Geometry check sheet. Reference: the model listing, model coordinates, mm. Face numbers are marked on the shaded views. A direction names the side the tool comes from. Give positions to 0.01 mm unless a question says otherwise; leave off trailing zeros. Write each loop counter-clockwise with the first axis right and the second up, starting at its lowest first coordinate (ties: lowest second). Pieces come first, ordered by that corner, then holes. Notation, with made-up numbers: (75, 72.25) - (117, 72.25) arc R27 cw to (117, 103.25) - close; hole circle Ø10 at (17, 81). An arc over 180 degrees is marked (long way). Write item = value, one per line. Start each with the question number.
(1) Section check B-B, the plane y = -12.85. Enter the section's corners in (x, z).
(2) Access from +Z, -Z, +X, -X, +Y, -Y to the whole of each face (thin tool, end or side, straight path). Record for the marked faces 1 and 2.
(3) Draft check along Y on the marked faces 3, 4 and 5. Enter one of: pulls with the +Y half, pulls with the -Y half, needs draft (parallel to the pull), parting line crosses it, or undercut.
(4) Thickness scan on L1, parallel to Y at x = 0, z = -0.95; L2, parallel to Z at x = 12, y = -9.5; L3, parallel to Y at x = 12.85, z = -1.2. Record the ranges inside material, lowest first.
(5) Section check C-C, the plane z = 5. Enter the section's corners in (x, y).
(6) Section check D-D, the plane y = 3.75. Enter the section's corners in (x, z), plus the area to 3 significant figures.
(7) Depth check by flat-ended pin: pin 1 Ø1.8 at (y, z) = (3, 2) entering from +X; pin 2 Ø5 at (y, z) = (-12.5, 3) entering from -X; pin 3 Ø1.5 at (y, z) = (-6, 3.5) entering from -X; pin 4 Ø2 at (y, z) = (1, 4) entering from -X. Enter the tip coordinate at first touch or a pass-through.
(8) Section check A-A, the plane x = 0. Enter the section's corners in (y, z).
```python
from build123d import *

# Parameters (mm, degrees)
F1_DEPTH = 2.5
F2_DEPTH = 7.5
F3_SIZE  = 0.5
F4_R     = 1.4
F5_DEPTH = 25


with BuildPart() as f1:
    # F0 (on Top) → F1 (new body)
    with BuildSketch(Plane.XY):
        with BuildLine():
            Line((11.83183, 11.514682), (8.85, 6.35))
            Line((8.85, 6.35), (8.85, 0))
            ThreePointArc((8.85, 0), (0, -8.85), (-8.85, 0))
            Line((-8.85, 0), (-8.85, 6.35))
            Line((-8.85, 6.35), (-11.83183, 11.514682))
            ThreePointArc((-11.83183, 11.514682), (0, -16.51), (11.83183, 11.514682))
        make_face()
        with BuildLine():
            Line((6.35, 2.019873), (6.35, 0))
            ThreePointArc((6.35, 0), (0, -6.35), (-6.35, 0))
            Line((-6.35, 0), (-6.35, 2.019873))
            Line((-6.35, 2.019873), (-8.85, 6.35))
            Line((-8.85, 6.35), (-8.85, 0))
            ThreePointArc((-8.85, 0), (0, -8.85), (8.85, 0))
            Line((8.85, 0), (8.85, 6.35))
            Line((8.85, 6.35), (6.35, 2.019873))
        make_face()
    extrude(amount=-F1_DEPTH)

    # F0 (on Top) → F2 (join)
    with BuildSketch(Plane.XY):
        with BuildLine():
            Line((6.35, 2.019873), (6.35, 0))
            ThreePointArc((6.35, 0), (0, -6.35), (-6.35, 0))
            Line((-6.35, 0), (-6.35, 2.019873))
            Line((-6.35, 2.019873), (-8.85, 6.35))
            Line((-8.85, 6.35), (-8.85, 0))
            ThreePointArc((-8.85, 0), (0, -8.85), (8.85, 0))
            Line((8.85, 0), (8.85, 6.35))
            Line((8.85, 6.35), (6.35, 2.019873))
        make_face()
    extrude(amount=F2_DEPTH)

    # F3
    f3_edges = [f1.edges().sort_by_distance(p)[0] for p in [
        (-8.85, 6.35, 3.75),
        (8.85, 6.35, 3.75),
    ]]
    chamfer(f3_edges, length=F3_SIZE)

    # F4 (on face) → F5 (cut)
    with BuildSketch(Plane.XY):
        with Locations((-12.85, 0)):
            Circle(F4_R)
        with Locations((12.85, 0)):
            Circle(F4_R)
        with Locations((0, -12.85)):
            Circle(F4_R)
    extrude(amount=-F5_DEPTH, mode=Mode.SUBTRACT)


solid = f1.part
```
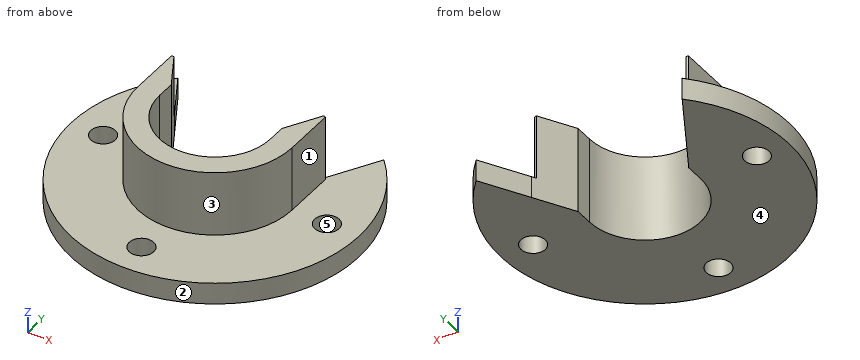
Model answer:
q1.outline = (-10.37, -2.5) - (-1.4, -2.5) - (-1.4, 0) - (-10.37, 0) - close; (1.4, -2.5) - (10.37, -2.5) - (10.37, 0) - (1.4, 0) - close
q2.face_1 = +Z, +X, +Y, -Y
q2.face_2 = +Z, -Z
q3.face_3 = pulls with the -Y half
q3.face_4 = needs draft
q3.face_5 = undercut
q4.L1 = -16.51 to -14.25, -11.45 to -6.35
q4.L2 = -2.5 to 0
q4.L3 = -10.37 to -1.4, 1.4 to 10.37
q5.outline = (-8.85, 0) arc R8.85 ccw to (8.85, 0) - (8.85, 5.85) - (8.6, 5.92) - (6.35, 2.02) - (6.35, 0) arc R6.35 cw to (-6.35, 0) - (-6.35, 2.02) - (-8.6, 5.92) - (-8.85, 5.85) - close
q6.outline = (-16.08, -2.5) - (-7.35, -2.5) - (-7.35, 7.5) - (-8.85, 7.5) - (-8.85, 0) - (-16.08, 0) - close; (7.35, -2.5) - (16.08, -2.5) - (16.08, 0) - (8.85, 0) - (8.85, 7.5) - (7.35, 7.5) - close
q6.area = 66.2 mm²
q7.pin_1 = 8.85
q7.pin_2 = through
q7.pin_3 = -7.12
q7.pin_4 = -8.85
q8.outline = (-16.51, -2.5) - (-14.25, -2.5) - (-14.25, 0) - (-16.51, 0) - close; (-11.45, -2.5) - (-6.35, -2.5) - (-6.35, 7.5) - (-8.85, 7.5) - (-8.85, 0) - (-11.45, 0) - close
